The model under review builds one solid part; all positions refer to its coordinate system, in mm. A direction names the side the tool comes from. Round coordinates to 2 decimals unless told otherwise and drop trailing zeros. Write each loop counter-clockwise with the first axis right and the second up, starting at its lowest first coordinate (ties: lowest second). Pieces come first, ordered by that corner, then holes. Notation, with made-up numbers: (7.25, 40.5) -> (16.25, 40.5) arc R15 ccw to (16.25, 54.5) -> close; hole circle Ø10 at (9.5, 80). An arc over 180 degrees is marked (long way). Use CSV: the item, a comma, the result in double quotes. Start each with the question number.
1) Wall thickness on probe 1 along Y at (x, z) = (-5, 4.8); probe 2 along Y at (x, z) = (6.5, 0.5); probe 3 along X at (y, z) = (-3, 4.25) (3 decimals): over which ranges is each line inside the solid? List them lowest first. Write a range as [from, to].
2) For pin 1 Ø1.5 at (x, y) = (4, -8) entering from +Z; pin 2 Ø0.9 at (x, z) = (-3.5, 0.5) entering from +Y; pin 3 Ø0.7 at (x, z) = (-4.5, 0.5) entering from -Y, all flat-tipped, find the tip position at first contact; note any pin that passes through.
3) Machinability: for faces 4 (the face through (-23.572, -15.994, 3.465)), 5 (the face through (-3.311, 22.245, 0.493)), 6 (the face through (10.5, -0.88, 3.46)), which of the approach directions +Z, -Z, +X, -X, +Y, -Y give a long, thin tool a straight path to every point of the face, cutting with its end or side? Answer none if there is none.
4) Mouldability with a two-part tool opening along X and no side actions: class faces 1 (the face through (-4, 22, 1)), 2 (the face through (4, -10, 0)), 3 (the face through (-5.6, 24.74, 3.46)) as released by +X, released by -X, zero draft, split by the parting line, or undercut.
5) Take a section at B-B, the plane z = 2. State how many separate pieces and enclosed holes the cut face has, then the cut area to 3 significant figures.
6) Take a section at A-A, the plane y = 4. Give the boundary of the cut face in (x, z) (3 decimals), then the cut area to 3 significant figures.
Autodesk Inventor part; units mm, degrees
ref_plane "Work Plane1" through (0, 0, 0) normal (0, 0, 1) x (1, 0, 0)
ref_plane "YZ Plane" through (0, 0, 0) normal (1, 0, 0) x (0, 1, 0)
ref_plane "XZ Plane" through (0, 0, 0) normal (0, 1, 0) x (-1, 0, 0)
sketch "Sketch1: base" plane through (0, 0, 0) normal (0, 0, 1) x (1, 0, 0)
  circle A0 centre (-5, 4) radius 16.25
  circle A1 centre (-5, 4) radius 20.75
  circle A2 centre (-21, -12) radius 4.75
  circle A3 centre (11, -12) radius 4.75
  line L0 (-21, -12) -> (11, -12) construction
  line L1 (-21, 20) -> (-21, -12) construction
  point P0 (0, 0)
  point P1 (-5, -12)
  point P2 (-21, 4)
  point P3 (-22.3145, -7.4355)
  point P4 (-16.4355, -13.3145)
  point P5 (6.4355, -13.3145)
  point P6 (12.3145, -7.4355)
  dimension "d0" = 9.5
  dimension "d1" = 32
  dimension "d2" = 41.5
  dimension "d3" = 32.5
  dimension "d4" = 32
sketch "Sketch2: tube stopper" plane through (0, 0, 0) normal (0, 0, 1) x (1, 0, 0)
  circle A0 centre (-5, 4) radius 14.875
  circle A1 centre (-5, 4) radius 16.25
  point P0 (0, 0)
  dimension "d14" = 29.75
extrude "Ex1: base" add sketch "Sketch1: base" along normal blind 6
ref_plane "Work Plane1" through (0, 0, 0) normal (0, 0, 1) x (1, 0, 0)
sketch "Sketch: text" plane through (0, 0, 0) normal (0, 0, -1) x (-1, 0, 0)
  line L0 (3.25, 24) -> (6.75, 24) construction
  line L1 (6.75, 24) -> (6.75, 20.5) construction
  line L2 (6.75, 20.5) -> (3.25, 20.5) construction
  line L3 (3.25, 20.5) -> (3.25, 24) construction
  line L4 (2.1748, 22.9624) -> (3.0901, 22.9624)
  line L5 (3.0901, 22.9624) -> (3.5386, 21.5071)
  line L6 (3.5386, 21.5071) -> (3.9993, 22.9624)
  line L7 (3.9993, 22.9624) -> (4.8871, 22.9624)
  line L8 (4.8871, 22.9624) -> (3.9108, 20.665)
  line L9 (3.9108, 20.665) -> (3.1297, 20.665)
  line L10 (3.1297, 20.665) -> (2.1748, 22.9624)
  line L11 (7.6056, 23.1211) -> (6.7299, 23.0143)
  spline S0 degree 2 poles (6.7299, 23.0143) (6.6964, 23.1973) (6.5347, 23.3499) (6.4157, 23.3499) knots 0 0 0 1 2 2 2
  spline S1 degree 2 poles (6.4157, 23.3499) (6.2021, 23.3499) (6.0831, 23.1333) knots 0 0 0 1 1 1
  spline S2 degree 2 poles (6.0831, 23.1333) (5.9946, 22.9777) (5.955, 22.4651) knots 0 0 0 1 1 1
  spline S3 degree 2 poles (5.955, 22.4651) (6.1136, 22.6268) (6.4462, 22.7794) (6.6628, 22.7794) knots 0 0 0 1 2 2 2
  spline S4 degree 2 poles (6.6628, 22.7794) (7.0869, 22.7794) (7.6727, 22.1753) (7.6727, 21.7084) knots 0 0 0 1 2 2 2
  spline S5 degree 2 poles (7.6727, 21.7084) (7.6727, 21.3942) (7.3767, 20.8755) (6.852, 20.6101) (6.4553, 20.6101) knots 0 0 0 1 2 3 3 3
  spline S6 degree 2 poles (6.4553, 20.6101) (5.9794, 20.6101) (5.4058, 20.9335) (5.061, 21.6474) (5.061, 22.2332) knots 0 0 0 1 2 3 3 3
  spline S7 degree 2 poles (5.061, 22.2332) (5.061, 23.0906) (5.7841, 23.8899) (6.4218, 23.8899) knots 0 0 0 1 2 2 2
  spline S8 degree 2 poles (6.4218, 23.8899) (6.8001, 23.8899) (7.2394, 23.716) (7.5293, 23.3773) (7.6056, 23.1211) knots 0 0 0 1 2 3 3 3
  spline S9 degree 2 poles (5.9855, 21.7084) (5.9855, 21.4522) (6.2448, 21.1593) (6.4309, 21.1593) knots 0 0 0 1 2 2 2
  spline S10 degree 2 poles (6.4309, 21.1593) (6.6048, 21.1593) (6.8367, 21.4217) (6.8367, 21.684) knots 0 0 0 1 2 2 2
  spline S11 degree 2 poles (6.8367, 21.684) (6.8367, 21.9525) (6.5957, 22.2332) (6.4157, 22.2332) knots 0 0 0 1 2 2 2
  spline S12 degree 2 poles (6.4157, 22.2332) (6.2326, 22.2332) (5.9855, 21.9617) (5.9855, 21.7084) knots 0 0 0 1 2 2 2
  point P0 (0, 0)
  point P1 (5, 4)
  point P2 (5, 20.5)
  dimension "d22" = 3.5
  dimension "d23" = 16.5
hole "Hole1: M3 heat-sets" at (11, -12, 0) at (-21, -12, 0) direction (0, 0, -1) diameter 4.2 end through all both
extrude "Ex: tube stopper" add sketch "Sketch2: tube stopper" along normal blind 1
fillet "Fillet1" radius 2 2 edges at (12.3145, -7.4355, 3) (-22.3145, -7.4355, 3)
fillet "Fillet2" radius 1 5 edges at (-23.1529, -7.0697, 0) (-23.6764, -15.9242, 0) (13.1529, -7.0697, 0) (13.6764, -15.9242, 0) (-5, 24.75, 0)
extrude "Ex: text" cut sketch "Sketch: text" against normal blind 1
properties part number "cage_inside_06"
Values found:
1,probe 1,"[-16.75, -12.25], [20.25, 24.75]"
1,probe 2,"[-13.27, -5.43], [13.43, 21.11]"
1,probe 3,"[-24.534, -19.665], [9.665, 14.534]"
2,pin 1,"z = 1"
2,pin 2,"y = 24.7"
2,pin 3,"y = -16.75"
3,face 4,"+Z, -Z"
3,face 5,"-Z"
3,face 6,"+Z"
4,face 1,"undercut"
4,face 2,"zero draft"
4,face 3,"split by the parting line"
5,separate pieces,"1"
5,enclosed holes,"3"
5,area,"605 mm²"
6,outline,"(-25.75, 1) arc R1 ccw to (-24.75, 0) -> (-19.875, 0) -> (-19.875, 1) -> (-21.25, 1) -> (-21.25, 6) -> (-25.75, 6) -> close; (9.875, 0) -> (14.75, 0) arc R1 ccw to (15.75, 1) -> (15.75, 6) -> (11.25, 6) -> (11.25, 1) -> (9.875, 1) -> close"
6,area,"56.3 mm²"
